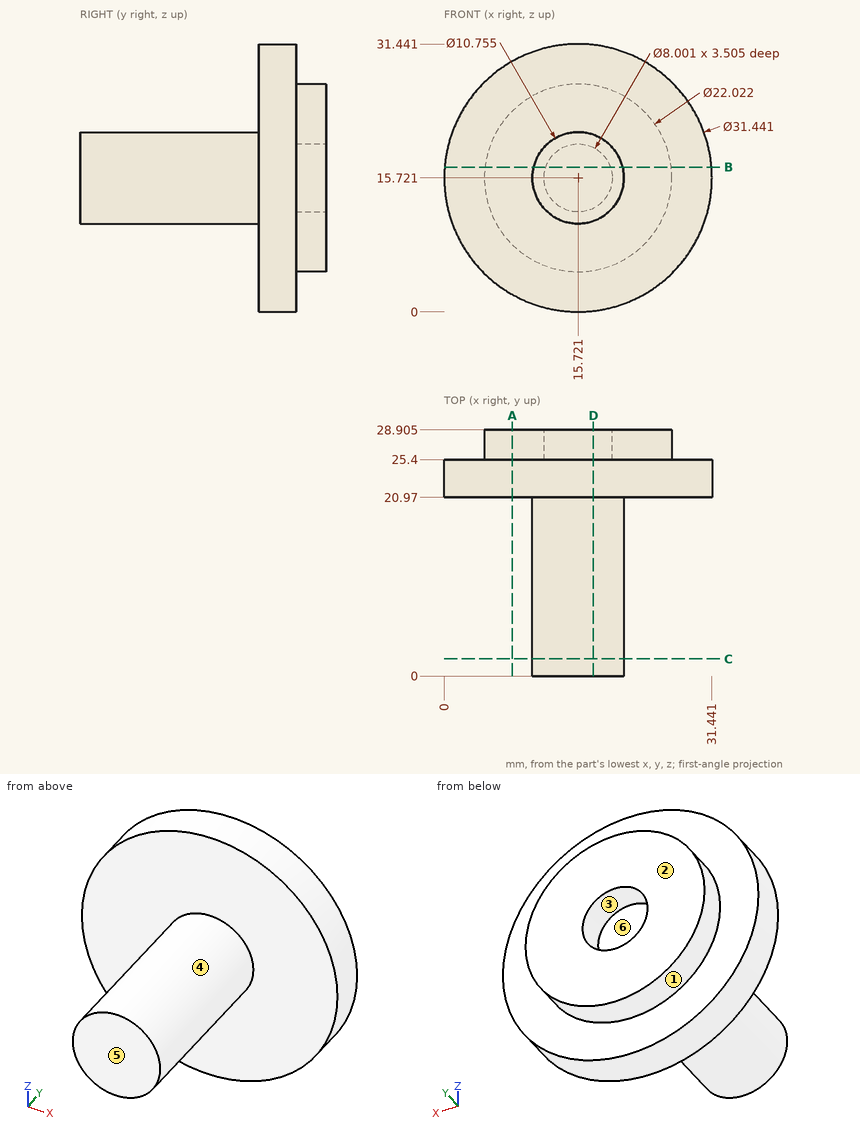
Design review of the part shown in the three views and the two pictorial views. Dimensions are in mm from the part's minimum x, y and z. A direction names the side the tool comes from. Give positions to 0.01 mm unless a question says otherwise; leave off trailing zeros. Loops run counter-clockwise (first coordinate to the right, second up) from the corner with the lowest first, then second, coordinate; pieces in that order, holes last. Notation, with made-up numbers: M -37,34.5 L 10,34.5 A10 cw 10,50.5 Z; hole C 57,33.5 d5. An arc over 180 degrees is marked long. Answer as a JSON object with one key per item and string values. Group by question number.
Q1. Add section C-C on y = 2. Give the boundary of the cut face in (x, z) (1 decimal).
Q2. Tool access review of the marked faces 4, 5 and 6: name each direction out of +Z, -Z, +X, -X, +Y, -Y from which nothing blocks a thin tool from reaching the whole face with its end or side.
Q3. For probe 1 along X at (y, z) = (5, 16); probe 2 along Y at (x, z) = (26.5, 20.5); probe 3 along Y at (x, z) = (16, 22) (1 decimal), list the stretches that pass through material, from the lowest coordinate up. Write a range as [from, to].
Q4. Mouldability with a two-part tool opening along X and no side actions: class the marked faces 1, 2 and 3 as +X half, -X half, draft (parallel to the pull), parting line (faces both ways), or undercut.
Q5. Insertion check: P1, Ø6, axis at y = 17, z = 26.5, coming from the -X side; P2, Ø10, axis at x = 21, y = 5, coming from the +Z side; P3, Ø1.5, axis at x = 21.5, z = 4, coming from the -Y side; P4, Ø10, axis at x = 24, y = 7.5, coming from the +Z side. Each pin has a flat end and moves straight along its axis. Give the tip position at first contact, or say it passes through.
Q6. Add section B-B on z = 17. Give the boundary of the cut face in (x, y) (1 decimal).
Q7. Add section D-D on x = 17.5. Give the boundary of the cut face in (y, z) (1 decimal).
Q8. Add section A-A on x = 8. Give the boundary of the cut face in (y, z) (1 decimal).
Checked values:
{
 "1": {"outline": "C 15.7,15.7 d10.8"},
 "2": {"face 4": "-Y", "face 5": "+Z, -Z, +X, -X, -Y", "face 6": "+Y"},
 "3": {"probe 1": "[10.35, 21.09]", "probe 2": "[20.97, 25.4]", "probe 3": "[21, 28.9]"},
 "4": {"face 1": "parting line", "face 2": "draft", "face 3": "undercut"},
 "5": {"P1": "through", "P2": "z = 21.09", "P3": "y = 20.97", "P4": "z = 19.98"},
 "6": {"outline": "M 0.1,21 L 10.5,21 L 10.5,0 L 20.9,0 L 20.9,21 L 31.4,21 L 31.4,25.4 L 26.7,25.4 L 26.7,28.9 L 19.5,28.9 L 19.5,25.4 L 11.9,25.4 L 11.9,28.9 L 4.8,28.9 L 4.8,25.4 L 0.1,25.4 Z"},
 "7": {"outline": "M 0,10.6 L 21,10.6 L 21,0.1 L 25.4,0.1 L 25.4,4.9 L 28.9,4.9 L 28.9,12.1 L 25.4,12.1 L 25.4,19.3 L 28.9,19.3 L 28.9,26.6 L 25.4,26.6 L 25.4,31.3 L 21,31.3 L 21,20.8 L 0,20.8 Z"},
 "8": {"outline": "M 21,2 L 25.4,2 L 25.4,7.9 L 28.9,7.9 L 28.9,23.6 L 25.4,23.6 L 25.4,29.4 L 21,29.4 Z"}
}
